Autodesk Inventor part; units mm, degrees
ref_plane "YZ Plane" through (0, 0, 0) normal (1, 0, 0) x (0, 1, 0)
ref_plane "XZ Plane" through (0, 0, 0) normal (0, 1, 0) x (-1, 0, 0)
ref_plane "XY Plane" through (0, 0, 0) normal (0, 0, 1) x (1, 0, 0)
sketch "Sketch5" plane through (0, 0, 0) normal (0, 0, 1) x (1, 0, 0)
  circle A0 centre (-16, 16) radius 1.75
  line L0 (-3.5516, 0) -> (2.966, 0)
  line L1 (0, 4.5757) -> (0, -5.4514)
  circle A1 centre (16, 16) radius 1.75
  circle A2 centre (-16, -16) radius 1.75
  circle A3 centre (16, -16) radius 1.75
  line L2 (19, -19) -> (-19, -19)
  line L3 (-19, -19) -> (-19, 19)
  line L4 (-19, 19) -> (19, 19)
  line L5 (19, 19) -> (19, -19)
  line L6 (19, -19) -> (-19, 19) construction
  line L7 (-19, -19) -> (19, 19) construction
  line L8 (4.0992, -12.7) -> (2.0496, -16.25)
  line L9 (2.0496, -16.25) -> (-2.0496, -16.25)
  line L10 (-2.0496, -16.25) -> (-4.0992, -12.7)
  line L11 (-4.0992, -12.7) -> (-2.0496, -9.15)
  line L12 (-2.0496, -9.15) -> (2.0496, -9.15)
  line L13 (2.0496, -9.15) -> (4.0992, -12.7)
  line L14 (4.0992, 12.7) -> (2.0496, 9.15)
  line L15 (2.0496, 9.15) -> (-2.0496, 9.15)
  line L16 (-2.0496, 9.15) -> (-4.0992, 12.7)
  line L17 (-4.0992, 12.7) -> (-2.0496, 16.25)
  line L18 (-2.0496, 16.25) -> (2.0496, 16.25)
  line L19 (2.0496, 16.25) -> (4.0992, 12.7)
  point P0 (0, 0)
  point P1 (0, 12.7)
  point P2 (0, -12.7)
  point P3 (0, -12.7)
  point P4 (0, 12.7)
  point P5 (0, -16.25)
  dimension "d47" = 3.5
  dimension "d50" = 32
  dimension "d53" = 32
  dimension "d56" = 16
  dimension "d57" = 16
  dimension "d58" = 38
  dimension "d59" = 38
  dimension "d73" = 7.1
  dimension "d74" = 7.1
extrude "Extrusion3" add sketch "Sketch5" along normal blind 5 contours L2 L3 L4 L5 | L8 L9 L10 L11 L12 L13 | L14 L15 L16 L17 L18 L19
sketch "Sketch6" plane through (0, 0, 5) normal (0, 0, 1) x (1, 0, 0)
  circle A0 centre (-16, 16) radius 1.75
  line L0 (-16, 19.4641) -> (-13, 17.7321)
  line L1 (-13, 17.7321) -> (-13, 14.2679)
  line L2 (-13, 14.2679) -> (-16, 12.5359)
  line L3 (-16, 12.5359) -> (-19, 14.2679)
  line L4 (-19, 14.2679) -> (-19, 17.7321)
  line L5 (-19, 17.7321) -> (-16, 19.4641)
  line L6 (0, 4.5757) -> (0, -5.4514)
  line L7 (-3.5516, 0) -> (2.966, 0)
  line L8 (16, 19.4641) -> (19, 17.7321)
  line L9 (19, 17.7321) -> (19, 14.2679)
  line L10 (19, 14.2679) -> (16, 12.5359)
  line L11 (16, 12.5359) -> (13, 14.2679)
  line L12 (13, 14.2679) -> (13, 17.7321)
  line L13 (13, 17.7321) -> (16, 19.4641)
  line L14 (-16, -12.5359) -> (-13, -14.2679)
  line L15 (-13, -14.2679) -> (-13, -17.7321)
  line L16 (-13, -17.7321) -> (-16, -19.4641)
  line L17 (-16, -19.4641) -> (-19, -17.7321)
  line L18 (-19, -17.7321) -> (-19, -14.2679)
  line L19 (-19, -14.2679) -> (-16, -12.5359)
  line L20 (16, -12.5359) -> (19, -14.2679)
  line L21 (19, -14.2679) -> (19, -17.7321)
  line L22 (19, -17.7321) -> (16, -19.4641)
  line L23 (16, -19.4641) -> (13, -17.7321)
  line L24 (13, -17.7321) -> (13, -14.2679)
  line L25 (13, -14.2679) -> (16, -12.5359)
  point P0 (0, 0)
  point P1 (-13, 16)
  point P2 (16, 16)
  point P3 (16, 16)
  point P4 (19, 16)
  point P5 (-16, -16)
  point P6 (-16, -16)
  point P7 (-13, -16)
  point P8 (16, -16)
  point P9 (16, -16)
  point P10 (19, -16)
  dimension "d62" = 6
  dimension "d65" = 32
  dimension "d68" = 32
extrude "Extrusion4" cut sketch "Sketch6" against normal blind 2.5
extrude "Extrusion5" cut sketch "Sketch5" along normal blind 3.2 contours L8 L9 L10 L11 L12 L13 | L14 L15 L16 L17 L18 L19
hole "Hole4" at (0, 12.7, 0) at (0, -12.7, 0) direction (0, 0, 1) diameter 4.2 end through all
sketch "Sketch7" plane through (0, 0, 5) normal (0, 0, 1) x (1, 0, 0)
  line L0 (-16.8038, -19) -> (-19, -17.7321)
  line L1 (-19, -19) -> (-19, 19)
  line L2 (19, -19) -> (-19, -19)
  line L3 (19, -19) -> (-19, 19) construction
  line L4 (-19, 17.7321) -> (-16.8038, 19)
  line L5 (-19, 19) -> (19, 19)
  line L6 (16.8038, 19) -> (19, 17.7321)
  line L7 (19, 19) -> (19, -19)
  line L8 (19, -17.7321) -> (16.8038, -19)
  point P0 (0, 0)
extrude "Extrusion6" cut sketch "Sketch7" against normal up to surface (2.5 mm away) contours L2 L1 L0 | L8 L7 L2 | L1 L5 L4 | L6 L5 L7
properties part number "RD-PDT-S-to-M4-bolts"
Can you work these out from the model? Positions are in its coordinate system, mm. A direction names the side the tool comes from. Coordinates: 2 decimals unless noted, no trailing zeros. Loops run counter-clockwise (first coordinate to the right, second up) from the corner with the lowest first, then second, coordinate; pieces in that order, holes last. Notation, with made-up numbers: M -2.75,80.25 L 35.25,80.25 A12 cw 35.25,94.25 Z; hole C 82,47.5 d6. An arc over 180 degrees is marked long. Return JSON: item names as keys, results as strings. Group by question number.
Item 1: If I drill on L1, parallel to Y at x = 0, z = 4.05; L2, parallel to Y at x = 16, z = 1.6; L3, parallel to X at y = 12.7, z = 4.1, over which ranges is the centre line in solid material (lowest first)? Write a range as from..to.
Item 2: Imagine slicing it at C-C (y = 17). Please give me the cut outline in (x, z).
Item 3: Imagine slicing it at A-A (z = 0.9). Please give me the cut outline in (x, y), and give its area (3 significant figures).
Item 4: Imagine slicing it at B-B (z = 4.15). Please give me the cut outline in (x, y), and give its area (3 significant figures).
Item 5: Thinking about a two-plate mould opening in X: for faces 1 (the flat face through (-16, 18, 2.5)), 2 (the flat face through (19, 0, 2)), 3 (the flat face through (-13, 16, 4)), which applies, released by +X, released by -X, zero draft, split by the parting line, or undercut?
Item 6: I'm going to push flat-ended pins straight in: pin 1 Ø3 at (x, y) = (16, -16) entering from -Z; pin 2 Ø2 at (y, z) = (-15.5, 4) entering from +X; pin 3 Ø4 at (x, y) = (-16, 16) entering from +Z. Where does each tip first touch, or does it pass through?
Item 7: On a 3-axis mill with a long thin cutter (end or side, diameter ignored), from which of +Z, -Z, +X, -X, +Y, -Y can I reach the whole of each face in a straight line? I mean faces 4 (the flat face through (17.5, -13.4, 3.8)), 5 (the flat face through (16, 18, 2.5)), 6 (the flat face through (14.113, -18.375, 3.768)), 7 (the flat face through (2, -11, 3.2)). Say none if no direction works.
Verdict:
{
 "1": {"L1": "y = -19..-14.8, -10.6..10.6, 14.8..19", "L2": "y = -19..-17.75, -14.25..14.25, 17.75..19", "L3": "x = -19..-16.28, -15.72..-2.1, 2.1..15.72, 16.28..19"},
 "2": {"outline": "M -19,0 L -17.44,0 L -17.44,2.5 L -19,2.5 Z; M -14.56,0 L 14.56,0 L 14.56,2.5 L 13,2.5 L 13,5 L -13,5 L -13,2.5 L -14.56,2.5 Z; M 17.44,0 L 19,0 L 19,2.5 L 17.44,2.5 Z"},
 "3": {"outline": "M -19,-19 L 19,-19 L 19,19 L -19,19 Z; hole C -16,-16 d3.5; hole C -16,16 d3.5; hole M -4.1,-12.7 L -2.05,-16.25 L 2.05,-16.25 L 4.1,-12.7 L 2.05,-9.15 L -2.05,-9.15 Z; hole M -4.1,12.7 L -2.05,9.15 L 2.05,9.15 L 4.1,12.7 L 2.05,16.25 L -2.05,16.25 Z; hole C 16,-16 d3.5; hole C 16,16 d3.5", "area": "1,320 mm^2"},
 "4": {"outline": "M -19,-14.27 L -16,-12.54 L -13,-14.27 L -13,-17.73 L -15.2,-19 L 15.2,-19 L 13,-17.73 L 13,-14.27 L 16,-12.54 L 19,-14.27 L 19,14.27 L 16,12.54 L 13,14.27 L 13,17.73 L 15.2,19 L -15.2,19 L -13,17.73 L -13,14.27 L -16,12.54 L -19,14.27 Z; hole C 0,-12.7 d4.2; hole C 0,12.7 d4.2", "area": "1,290 mm^2"},
 "5": {"face 1": "undercut", "face 2": "released by +X", "face 3": "released by -X"},
 "6": {"pin 1": "passes through", "pin 2": "stops at x = 13", "pin 3": "stops at z = 2.5"},
 "7": {"face 4": "+Z, -Y", "face 5": "+Z", "face 6": "+Z, +X", "face 7": "-Z"}
}
